Can you work these out from the model? Positions are in its coordinate system, mm. Face numbers are marked on the shaded views. A direction names the side the tool comes from. Give positions to 0.01 mm unless a question says otherwise; leave off trailing zeros. Loops run counter-clockwise (first coordinate to the right, second up) from the corner with the lowest first, then second, coordinate; pieces in that order, holes last. Notation, with made-up numbers: M 6.5,21.5 L 48.5,21.5 A19 ccw 48.5,31.5 Z; hole C 81.5,89 d1. An arc over 180 degrees is marked long. Answer as a JSON object with one key per item and string values.
Autodesk Fusion 360 part; units mm, degrees
sketch "Sketch1" plane through (0, 0, 0) normal (0, 1, 0) x (1, 0, 0)
  line L0 (35, -15) -> (-35, -15)
  line L1 (-35, -15) -> (-35, 15)
  line L2 (-35, 15) -> (35, 15)
  line L3 (35, 15) -> (35, -15)
  line L4 (35, -15) -> (-35, 15) construction
  line L5 (-35, -15) -> (35, 15) construction
  line L6 (-30, 10) -> (30, 10)
  line L7 (30, 10) -> (30, -10)
  line L8 (30, -10) -> (-30, -10)
  line L9 (-30, -10) -> (-30, 10)
  dimension "d1" = 70
  dimension "d2" = 30
  dimension "d3" = 5
extrude "Extrude1" add sketch "Sketch1" along normal mid plane 30
sketch "Sketch2" plane through (35, 0, 0) normal (1, 0, 0) x (0, 1, 0)
  line L0 (-15, -15) -> (15, -15)
  line L1 (15, -15) -> (15, 15)
  line L2 (15, 15) -> (-15, 15)
  line L3 (-15, 15) -> (-15, -15)
  circle A0 centre (-10, -2.5) radius 1.6
  dimension "d6" = 3.2
  dimension "d7" = 12.5
  dimension "d8" = 5
extrude "Extrude2" cut sketch "Sketch2" against normal blind 76 contours A0
sketch "Sketch3" plane through (0, 0, 15) normal (0, 0, 1) x (-1, 0, 0)
  line L0 (-35, 15) -> (-35, -15)
  line L1 (-35, -15) -> (35, -15)
  line L2 (35, -15) -> (35, 15)
  line L3 (35, 15) -> (-35, 15)
  circle A0 centre (0, 0) radius 1.6
  dimension "d11" = 3.2
extrude "Extrude3" cut sketch "Sketch3" against normal blind 41 contours A0
equation "d7 = ( 25 / 2 ) * 1 mm"
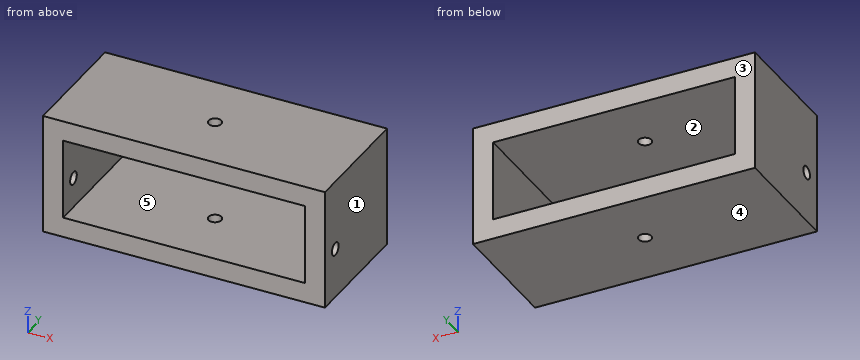
1) Suppose I cut it at C-C, the plane y = 0. Write out the boundary of the cut face in (x, z), and give its area (3 significant figures).
Answer list:
{"outline": "M -35,-15 L -1.6,-15 L -1.6,-10 L -30,-10 L -30,10 L -1.6,10 L -1.6,15 L -35,15 Z; M 1.6,-15 L 35,-15 L 35,15 L 1.6,15 L 1.6,10 L 30,10 L 30,-10 L 1.6,-10 Z", "area": "868 mm^2"}
2) Please list where these lines run through material, in increasing order: line 1 along Z through (x, y) = (23.5, 3); line 2 along Z through (x, y) = (-32.35, -10); line 3 along X through (y, z) = (4, 0.5). Write a range as from..to.
Answer list:
{"line 1": "-15..-10, 10..15", "line 2": "-15..-4.1, -0.9..15", "line 3": "-35..-30, 30..35"}
3) Suppose I cut it at B-B, the plane z = -2.5. Write out the boundary of the cut face in (x, y).
Answer list:
{"outline": "M -35,-15 L -30,-15 L -30,-11.6 L -35,-11.6 Z; M -35,-8.4 L -30,-8.4 L -30,15 L -35,15 Z; M 30,-15 L 35,-15 L 35,-11.6 L 30,-11.6 Z; M 30,-8.4 L 35,-8.4 L 35,15 L 30,15 Z"}
4) If we mould it in two halves opening along X, with no side actions, what happens to the marked faces 1, 2 and 3? For each: +X half, -X half, draft (parallel to the pull), parting line (faces both ways), or undercut.
Answer list:
{"face 1": "+X half", "face 2": "undercut", "face 3": "draft"}
5) For the marked faces 4 and 5, which set-ups out of +Z, -Z, +X, -X, +Y, -Y let a thin tool reach every point of the face, with its end or its side?
Answer list:
{"face 4": "-Z, +X, -X, +Y, -Y", "face 5": "+Y, -Y"}
6) Suppose I cut it at D-D, the plane x = 0. Write out the boundary of the cut face in (y, z), and give its area (3 significant figures).
Answer list:
{"outline": "M -15,-15 L -1.6,-15 L -1.6,-10 L -15,-10 Z; M -15,10 L -1.6,10 L -1.6,15 L -15,15 Z; M 1.6,-15 L 15,-15 L 15,-10 L 1.6,-10 Z; M 1.6,10 L 15,10 L 15,15 L 1.6,15 Z", "area": "268 mm^2"}
7) Suppose I cut it at A-A, the plane x = 16.5. Write out the boundary of the cut face in (y, z).
Answer list:
{"outline": "M -15,-15 L 15,-15 L 15,-10 L -15,-10 Z; M -15,10 L 15,10 L 15,15 L -15,15 Z"}
